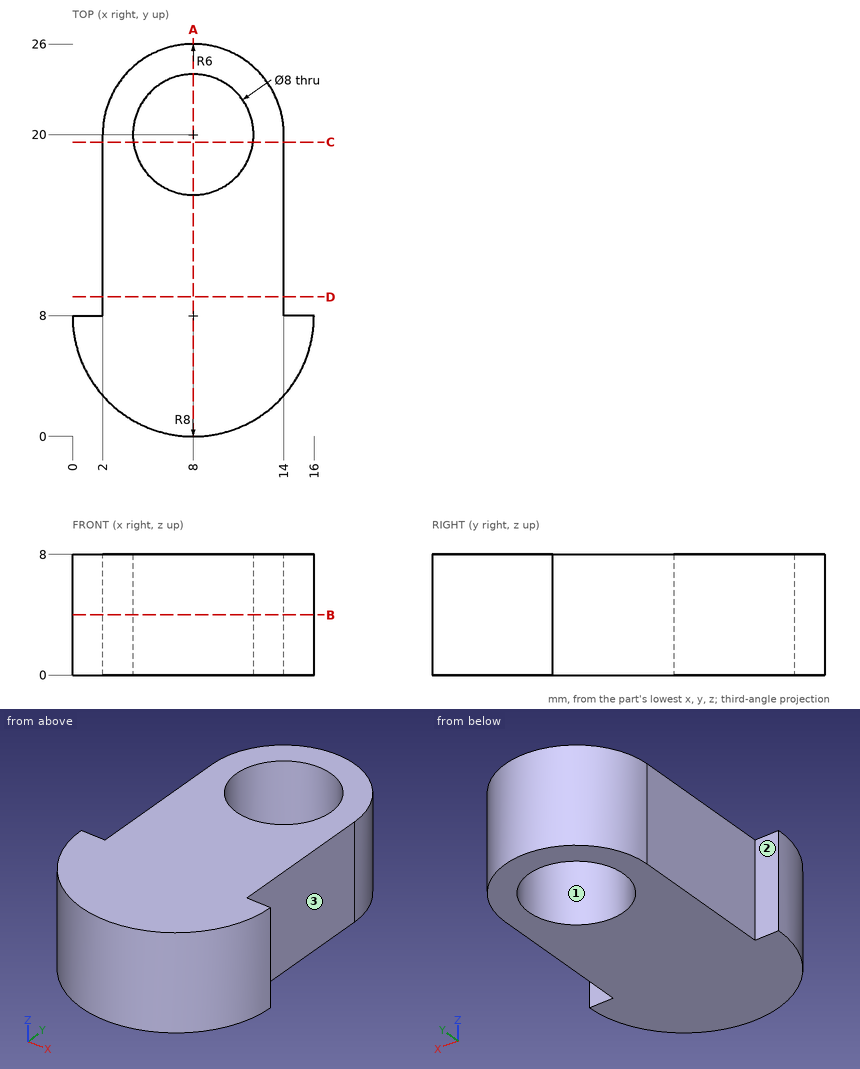
Print and shaded views of the part. All mm, measured from the part's lowest x, y and z. A direction names the side the tool comes from. Coordinates: 2 decimals unless noted, no trailing zeros. Order: outer loops, then holes, each group sorted by start corner. A loop starts at its lowest first (then second) coordinate and runs counter-clockwise, first axis right, second up. Notation, with made-up numbers: M 69.5,-37.5 L 102.5,-37.5 A16 ccw 102.5,-11.5 Z; hole C 26,-8 d8. An arc over 180 degrees is marked long. Answer as CSV lines item,"result".
1) 3-axis set-ups, long thin cutter, end or side, ignore diameter. For the marked faces 1, 2 and 3: which of +Z, -Z, +X, -X, +Y, -Y reach the whole face in a straight line?
Verdict:
face 1,"+Z, -Z"
face 2,"+Z, -Z, -X, +Y"
face 3,"+Z, -Z, +X, +Y"
2) Cut at C-C (y = 19.5). List the corners of the cut face in (x, z), then the cut area to 3 significant figures.
Verdict:
outline,"M 2,0 L 4.03,0 L 4.03,8 L 2,8 Z; M 11.97,0 L 14,0 L 14,8 L 11.97,8 Z"
area,"32.5 mm2"
3) Cut at D-D (y = 9.25). List the corners of the cut face in (x, z), then the cut area to 3 significant figures.
Verdict:
outline,"M 2,0 L 14,0 L 14,8 L 2,8 Z"
area,"96.0 mm2"
4) Cut at B-B (z = 4). List the corners of the cut face in (x, y).
Verdict:
outline,"M 0,8 A8 ccw 16,8 L 14,8 L 14,20 A6 ccw 2,20 L 2,8 Z; hole C 8,20 d8"
5) Cut at A-A (x = 8). List the corners of the cut face in (y, z), then the cut area to 3 significant figures.
Verdict:
outline,"M 0,0 L 16,0 L 16,8 L 0,8 Z; M 24,0 L 26,0 L 26,8 L 24,8 Z"
area,"144 mm2"
6) Flat gauge pins, fed straight in: P1, Ø4, axis at y = 12.5, z = 2.5, coming from the -X side; P2, Ø1, axis at x = 15, z = 3.5, coming from the +Y side; P3, Ø4, axis at y = 3.5, z = 3, coming from the -X side. Where does each tip first touch, or does it go through?
Verdict:
P1,"x = 2"
P2,"y = 8"
P3,"x = 0.4"
7) Drill centre lines: L1, parallel to Y at x = 8, z = 5.25; L2, parallel to X at y = 19, z = 7; L3, parallel to Y at x = 6.5, z = 6. Where is each one in solid material? Low to high. Write a range as from..to.
Verdict:
L1,"0..16, 24..26"
L2,"2..4.13, 11.87..14"
L3,"0.14..16.29, 23.71..25.81"
